Build history of the part. All positions in model axes, mm. A direction names the side the tool comes from. Coordinates: 2 decimals unless noted, no trailing zeros. Write each loop counter-clockwise with the first axis right and the second up, starting at its lowest first coordinate (ties: lowest second). Pieces come first, ordered by that corner, then holes.
```python
from build123d import *

# Parameters (mm, degrees)
F0_W          = 25.4
F0_H          = 38.1
F1_DEPTH      = 5
F2_DEPTH      = 50.8
F3_W          = 25.4
F3_H          = 38.1
F4_DEPTH      = 5
F5_R          = 2
F6_DEPTH      = 50.801
F6_DEPTH_BACK = 50.801
F8_R          = 5
F9_DEPTH      = 33.1


with BuildPart() as f1:
    # F0 (on Front) → F1 (new body)
    with BuildSketch(Plane.XZ):
        Polygon((-12.7, 63.5), (-50.8, 63.5), (-12.7, 25.4), align=None)
        with Locations((0, 44.45)):
            Rectangle(F0_W, F0_H)
        Polygon((12.7, 63.5), (12.7, 25.4), (50.8, 63.5), align=None)
    extrude(amount=F1_DEPTH)

    # F0 (on Front) → F2 (join)
    with BuildSketch(Plane.XZ):
        Polygon((12.7, 63.5), (12.7, 25.4), (50.8, 63.5), align=None)
        Polygon((-12.7, 63.5), (-50.8, 63.5), (-12.7, 25.4), align=None)
    extrude(amount=-F2_DEPTH)

    # F3 (on face) → F4 (join)
    with BuildSketch(Plane(origin=(0, 50.8, 0), x_dir=(-1, 0, 0), z_dir=(0, 1, 0))):
        Polygon((50.8, 63.5), (12.7, 63.5), (12.7, 25.4), align=None)
        with Locations((0, 44.45)):
            Rectangle(F3_W, F3_H)
        Polygon((-12.7, 25.4), (-12.7, 63.5), (-50.8, 63.5), align=None)
    extrude(amount=F4_DEPTH)

    # F5 (on Right) → F6 (cut, two sides)
    with BuildSketch(Plane.YZ) as f6_sk:
        with Locations((38.1, 34.925)):
            Circle(F5_R)
        with Locations((12.7, 34.925)):
            Circle(F5_R)
    extrude(amount=-F6_DEPTH, mode=Mode.SUBTRACT)
    extrude(f6_sk.sketch, amount=F6_DEPTH_BACK, mode=Mode.SUBTRACT)

    # F8 (on offset) → F9 (cut, through all)
    with BuildSketch(Plane.YZ.offset(50.8)):
        with Locations((38.1, 34.925)):
            Circle(F8_R)
        with Locations((12.7, 34.925)):
            Circle(F8_R)
    extrude(amount=-F9_DEPTH, mode=Mode.SUBTRACT)


solid = f1.part
```
1. Mould opens along X. For faces 1 (the face through (17.7, 15, 35)), 2 (the face through (15.16, 39.18, 36.61)), 3 (the face through (0, 0, 45)) say: +X half, -X half, draft (parallel to the pull), parting line (faces both ways), or undercut.
Computed values:
face 1: +X half
face 2: draft
face 3: undercut
2. Flat gauge pins, fed straight in: pin 1 (3 mm diameter, centred on y = 12.7, z = 34.925, fed in from +X); pin 2 (6.5 mm diameter, centred on y = 38.1, z = 34.925, fed in from -X) (3 decimals); pin 3 (3 mm diameter, centred on y = 37.5, z = 34, fed in from +X); pin 4 (8 mm diameter, centred on y = 14.5, z = 40.5, fed in from +X). Where does each tip first touch, or does it go through?
Computed values:
pin 1: passes through
pin 2: stops at x = -25.475
pin 3: stops at x = 17.7
pin 4: stops at x = 31.8
3. Saw through at D-D on y = 3. List the corners of the cut face in (x, z), plus the area to 3 significant figures.
Computed values:
outline: (-50.8, 63.5) - (-12.7, 25.4) - (-12.7, 63.5) - close; (12.7, 25.4) - (50.8, 63.5) - (12.7, 63.5) - close
area: 1,450 mm2
4. Probe line 1 along Y through (x, z) = (-2, 52); line 2 along X through (y, z) = (9, 50); line 3 along X through (y, z) = (25, 45). List the from-to ranges inside material, lowest first.
Computed values:
line 1: y = -5 to 0, 50.8 to 55.8
line 2: x = -37.3 to -12.7, 12.7 to 37.3
line 3: x = -32.3 to -12.7, 12.7 to 32.3
5. Saw through at A-A on x = 9. List the corners of the cut face in (y, z), plus the area to 3 significant figures.
Computed values:
outline: (-5, 25.4) - (0, 25.4) - (0, 63.5) - (-5, 63.5) - close; (50.8, 25.4) - (55.8, 25.4) - (55.8, 63.5) - (50.8, 63.5) - close
area: 381 mm2
6. 3-axis set-ups, long thin cutter, end or side, ignore diameter. For faces 4 (the face through (0, 53, 25.4)), 5 (the face through (21.48, 38.29, 39.92)), 6 (the face through (12.7, 25, 45)): which of +Z, -Z, +X, -X, +Y, -Y reach the whole face in a straight line?
Computed values:
face 4: -Z, +X, -X, +Y, -Y
face 5: +X
face 6: +Z, -Z
7. Saw through at C-C on z = 52. List the corners of the cut face in (x, y), plus the area to 3 significant figures.
Computed values:
outline: (-39.3, -5) - (39.3, -5) - (39.3, 55.8) - (-39.3, 55.8) - close; hole (-12.7, 0) - (12.7, 0) - (12.7, 50.8) - (-12.7, 50.8) - close
area: 3,490 mm2
8. Saw through at B-B on y = 38.1. List the corners of the cut face in (x, z) (3 decimals), plus the area to 3 significant figures.
Computed values:
outline: (-50.8, 63.5) - (-24.225, 36.925) - (-12.7, 36.925) - (-12.7, 63.5) - close; (-20.225, 32.925) - (-12.7, 25.4) - (-12.7, 32.925) - close; (12.7, 25.4) - (17.7, 30.4) - (17.7, 32.925) - (12.7, 32.925) - close; (12.7, 36.925) - (17.7, 36.925) - (17.7, 39.925) - (27.225, 39.925) - (50.8, 63.5) - (12.7, 63.5) - close
area: 1,350 mm2
